```python
from build123d import *

# Parameters (mm, degrees)
F0_R     = 9.525
F0_W     = 12.7
F0_H     = 50.8
F1_DEPTH = 12.7
F2_W     = 12.7
F2_H     = 50.8
F3_DEPTH = 12.7
F4_W     = 12.7
F4_H     = 50.8
F5_DEPTH = 12.7
F6_R     = 12.7
F7_DEPTH = 76.2


with BuildPart() as f1:
    # F0 (on Front) → F1 (new body, symmetric)
    with BuildSketch(Plane.XZ):
        with BuildLine():
            ThreePointArc((0, -25.4), (17.960512, -17.960512), (25.4, 0))
            ThreePointArc((25.4, 0), (17.960512, 17.960512), (0, 25.4))
            ThreePointArc((0, 25.4), (-25.4, 0), (0, -25.4))
        make_face()
        Circle(F0_R, mode=Mode.SUBTRACT)
        with BuildLine():
            ThreePointArc((0, 25.4), (17.960512, 17.960512), (25.4, 0))
            ThreePointArc((25.4, 0), (17.960512, -17.960512), (0, -25.4))
            Line((0, -25.4), (38.1, -25.4))
            Line((38.1, -25.4), (38.1, 25.4))
            Line((38.1, 25.4), (0, 25.4))
        make_face()
        with Locations((44.45, 0)):
            Rectangle(F0_W, F0_H)
    extrude(amount=F1_DEPTH, both=True)

    # F2 (on face) → F3 (join)
    with BuildSketch(Plane.XZ.offset(12.7)):
        with Locations((44.45, 0)):
            Rectangle(F2_W, F2_H)
    extrude(amount=F3_DEPTH)

    # F4 (on face) → F5 (join)
    with BuildSketch(Plane(origin=(0, 12.7, 0), x_dir=(-1, 0, 0), z_dir=(0, 1, 0))):
        with Locations((-44.45, 0)):
            Rectangle(F4_W, F4_H)
    extrude(amount=F5_DEPTH)

    # F6 (on face) → F7 (join)
    with BuildSketch(Plane.YZ.offset(50.8)):
        Circle(F6_R)
    extrude(amount=F7_DEPTH)


solid = f1.part
```
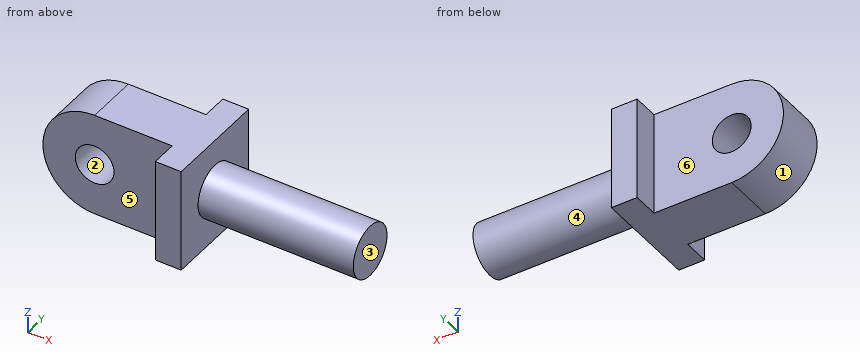
Part model, mm, in its own coordinate system. Face numbers are marked on the shaded views. A direction names the side the tool comes from. Round coordinates to 2 decimals unless told otherwise and drop trailing zeros. Loops run counter-clockwise (first coordinate to the right, second up) from the corner with the lowest first, then second, coordinate; pieces in that order, holes last.
Item 1: Mould opens along Z. For the marked faces 1, 2 and 3 say: +Z half, -Z half, draft (parallel to the pull), parting line (faces both ways), or undercut.
Item 2: Drill centre lines: line 1 (Y direction, x = 30, z = -19.5); line 2 (X direction, y = 19.5, z = 16); line 3 (X direction, y = -1, z = -7.5). Where is each one in solid material? Low to high.
Item 3: Cut at B-B, the plane y = 0. Give the cut face in (x, z) (3 decimals), then the cut area to 3 significant figures.
Item 4: Cut at A-A, the plane z = 0. Give the cut face in (x, y) (3 decimals), then the cut area to 3 significant figures.
Item 5: Drop flat-ended pins along their axis: P1, Ø22, axis at x = 0, z = 0, coming from the -Y side; P2, Ø3, axis at y = -9.5, z = 17, coming from the -X side; P3, Ø4, axis at y = 21.5, z = 3, coming from the -X side. Give the stop position or say it passes through.
Item 6: 3-axis set-ups, long thin cutter, end or side, ignore diameter. For the marked faces 4, 5 and 6: which of +Z, -Z, +X, -X, +Y, -Y reach the whole face in a straight line?
Item 7: Cut at C-C, the plane x = -2.5. Give the cut face in (y, z), then the cut area to 3 significant figures.
Item 8: Cut at D-D, the plane z = -21.5. Give the cut face in (x, y), then the cut area to 3 significant figures.
A:
1. face 1: parting line
1. face 2: undercut
1. face 3: draft
2. line 1: y = -12.7 to 12.7
2. line 2: x = 38.1 to 50.8
2. line 3: x = -24.27 to -5.87, 5.87 to 127
3. outline: (0, -25.4) - (50.8, -25.4) - (50.8, -12.7) - (127, -12.7) - (127, 12.7) - (50.8, 12.7) - (50.8, 25.4) - (0, 25.4) arc R25.4 ccw to start; hole circle Ø19.05 at (0, 0)
3. area: 5,240 mm2
4. outline: (-25.4, -12.7) - (-9.525, -12.7) - (-9.525, 12.7) - (-25.4, 12.7) - close; (9.525, -12.7) - (38.1, -12.7) - (38.1, -25.4) - (50.8, -25.4) - (50.8, -12.7) - (127, -12.7) - (127, 12.7) - (50.8, 12.7) - (50.8, 25.4) - (38.1, 25.4) - (38.1, 12.7) - (9.525, 12.7) - close
4. area: 3,710 mm2
5. P1: stops at y = -12.7
5. P2: stops at x = -20.12
5. P3: stops at x = 38.1
6. face 4: +X
6. face 5: +Z, -Z, -X, -Y
6. face 6: +Z, -Z, -X, +Y
7. outline: (-12.7, -25.28) - (12.7, -25.28) - (12.7, -9.19) - (-12.7, -9.19) - close; (-12.7, 9.19) - (12.7, 9.19) - (12.7, 25.28) - (-12.7, 25.28) - close
7. area: 817 mm2
8. outline: (-13.52, -12.7) - (38.1, -12.7) - (38.1, -25.4) - (50.8, -25.4) - (50.8, 25.4) - (38.1, 25.4) - (38.1, 12.7) - (-13.52, 12.7) - close
8. area: 1,960 mm2
